Part model, mm, in its own coordinate system. A direction names the side the tool comes from. Round coordinates to 2 decimals unless told otherwise and drop trailing zeros. Loops run counter-clockwise (first coordinate to the right, second up) from the corner with the lowest first, then second, coordinate; pieces in that order, holes last.
1) Probe line 1 (Y direction, x = -0.25, z = 2); line 2 (Y direction, x = 0, z = 21.5); line 3 (X direction, y = -10, z = 1.15). List the from-to ranges inside material, lowest first.
2) 3-axis set-ups, long thin cutter, end or side, ignore diameter. For faces 1 (the cylindrical face through (-5.287, 5.248, 14.154)), 2 (the cylindrical face through (5.287, -5.248, 14.154)), 3 (the flat face through (-6, 0, 14)), 4 (the cylindrical face through (5.248, 5.287, 14.154)): which of +Z, -Z, +X, -X, +Y, -Y reach the whole face in a straight line?
3) Drop flat-ended pins along their axis: P1, Ø3, axis at x = 5.5, z = 10, coming from the +Y side; P2, Ø1.5, axis at x = -3.5, z = 17.5, coming from the -Y side; P3, Ø7.5, axis at x = 0, z = 13, coming from the +Y side. Give the stop position or say it passes through.
4) Mould opens along X. For faces 5 (the flat face through (0, 0, 15.9)), 6 (the cylindrical face through (-2.8, 0.1, 20.5)), 7 (the flat face through (6, 0, 14)), 8 (the flat face through (0, 6, 14)) say: +X half, -X half, draft (parallel to the pull), parting line (faces both ways), or undercut.
5) Band-saw the part on C-C, the plane z = 21.25. Write the cut outline in (x, y).
6) Band-saw the part on D-D, the plane y = 0. Write the cut outline in (x, z).
7) Band-saw the part on B-B, the plane x = 0. Write the cut outline in (y, z).
8) Band-saw the part on A-A, the plane y = 10. Write the cut outline in (x, z), then the cut area to 3 significant figures.
from build123d import *

# Parameters (mm, degrees)
ESQUISSE1_W             = 20
ESQUISSE1_H             = 30
ESQUISSE1_R             = 2.1
BOSS_EXTRU_1_DEPTH      = 3
ESQUISSE2_W             = 12
ESQUISSE2_H             = 12
BOSS_EXTRU_2_DEPTH      = 22
ESQUISSE3_OUTSIDE_W     = 30.774
ESQUISSE3_OUTSIDE_H     = 40.774
ESQUISSE3_OUTSIDE_W_2   = 12
ESQUISSE3_OUTSIDE_H_2   = 12
ESQUISSE3_OUTSIDE_R     = 2.8
ENL_V_MAT_EXTRU_1_DEPTH = 9.1
CONG_1_R                = 2.5


with BuildPart() as part:
    # Esquisse1 → Boss.-Extru.1 (new body)
    with BuildSketch(Plane.XY):
        Rectangle(ESQUISSE1_W, ESQUISSE1_H)
        with Locations((0, 10)):
            Circle(ESQUISSE1_R, mode=Mode.SUBTRACT)
        with Locations(Location((0, -10, 0), (0, 0, 180))):
            Circle(ESQUISSE1_R, mode=Mode.SUBTRACT)
    extrude(amount=BOSS_EXTRU_1_DEPTH)

    # Esquisse2 → Boss.-Extru.2 (add)
    with BuildSketch(Plane.XY.offset(3)):
        Rectangle(ESQUISSE2_W, ESQUISSE2_H)
    extrude(amount=BOSS_EXTRU_2_DEPTH)

    # Esquisse3 outside → Enlèv. mat.-Extru.1 (cut)
    # profile 1 of 2: a face of its own
    with BuildSketch(Plane.XY.offset(25)):
        Rectangle(ESQUISSE3_OUTSIDE_W, ESQUISSE3_OUTSIDE_H)
        Rectangle(ESQUISSE3_OUTSIDE_W_2, ESQUISSE3_OUTSIDE_H_2, mode=Mode.SUBTRACT)
    # profile 2 of 2: a face of its own
    with BuildSketch(Plane.XY.offset(25)):
        Circle(ESQUISSE3_OUTSIDE_R)
    extrude(amount=-ENL_V_MAT_EXTRU_1_DEPTH, mode=Mode.SUBTRACT)

    # Congé1
    cong_1_edges = [part.edges().sort_by_distance(p)[0] for p in [
        (-6, 6, 14),
        (-6, -6, 14),
        (6, -6, 14),
        (6, 6, 14),
        (-10, 15, 1.5),
        (10, 15, 1.5),
        (10, -15, 1.5),
        (-10, -15, 1.5),
    ]]
    fillet(cong_1_edges, radius=CONG_1_R)


solid = part.part
Reported:
1. line 1: y = -15 to -12.09, -7.91 to 7.91, 12.09 to 15
1. line 2: y = -6 to -2.8, 2.8 to 6
1. line 3: x = -10 to -2.1, 2.1 to 10
2. face 1: +Z, -X, +Y
2. face 2: +Z, +X, -Y
2. face 3: +Z, -X, +Y, -Y
2. face 4: +Z, +X, +Y
3. P1: stops at y = 5.95
3. P2: stops at y = -6
3. P3: stops at y = 6
4. face 5: undercut
4. face 6: undercut
4. face 7: +X half
4. face 8: draft
5. outline: (-6, -3.5) arc R2.5 ccw to (-3.5, -6) - (3.5, -6) arc R2.5 ccw to (6, -3.5) - (6, 3.5) arc R2.5 ccw to (3.5, 6) - (-3.5, 6) arc R2.5 ccw to (-6, 3.5) - close; hole circle Ø5.6 at (0, 0)
6. outline: (-10, 0) - (10, 0) - (10, 3) - (6, 3) - (6, 25) - (2.8, 25) - (2.8, 15.9) - (-2.8, 15.9) - (-2.8, 25) - (-6, 25) - (-6, 3) - (-10, 3) - close
7. outline: (-15, 0) - (-12.1, 0) - (-12.1, 3) - (-15, 3) - close; (-7.9, 0) - (7.9, 0) - (7.9, 3) - (6, 3) - (6, 25) - (2.8, 25) - (2.8, 15.9) - (-2.8, 15.9) - (-2.8, 25) - (-6, 25) - (-6, 3) - (-7.9, 3) - close; (12.1, 0) - (15, 0) - (15, 3) - (12.1, 3) - close
8. outline: (-10, 0) - (-2.1, 0) - (-2.1, 3) - (-10, 3) - close; (2.1, 0) - (10, 0) - (10, 3) - (2.1, 3) - close
8. area: 47.4 mm2
